Could you check a few things on this drawing? It's one solid part, dimensions in mm from its lowest x, y, z. Give positions to 0.01 mm unless a question says otherwise; leave off trailing zeros. Loops run counter-clockwise (first coordinate to the right, second up) from the corner with the lowest first, then second, coordinate; pieces in that order, holes last. Notation, with made-up numbers: (70, 15.25) - (118, 15.25) arc R32 ccw to (118, 45.25) - close; hole circle Ø1 at (86, -8). An arc over 180 degrees is marked (long way). Return JSON: item names as keys, results as strings. Group by question number.
(1) If we section it at B-B (x = 30): Please give me the cut outline in (y, z), then the cut area to 3 significant figures.
(2) If we mould it in two halves opening along Z, with no side actions, what happens to the marked faces 1, 2 and 3? For each: released by +Z, released by -Z, zero draft, split by the parting line, or undercut.
(3) I need wall thicknesses on probe 1 along Z at (x, y) = (118.5, 24); probe 2 along X at (y, z) = (9.25, 6.5) (1 decimal). Which ranges of each line are inside material? Lowest first, please. Write a range as [from, to].
(4) For P1, Ø6.5, axis at x = 74, y = 8.5, coming from the -Z side, with a flat end and sliding along its axis, tell me the tip position at first contact or that it passes through.
(5) If we section it at C-C (x = 69.85): State how many separate pieces and enclosed holes the cut face has, then the cut area to 3 significant figures.
(6) If we section it at A-A (z = 115.5): Please give me the cut outline in (x, y), then the cut area to 3 significant figures.
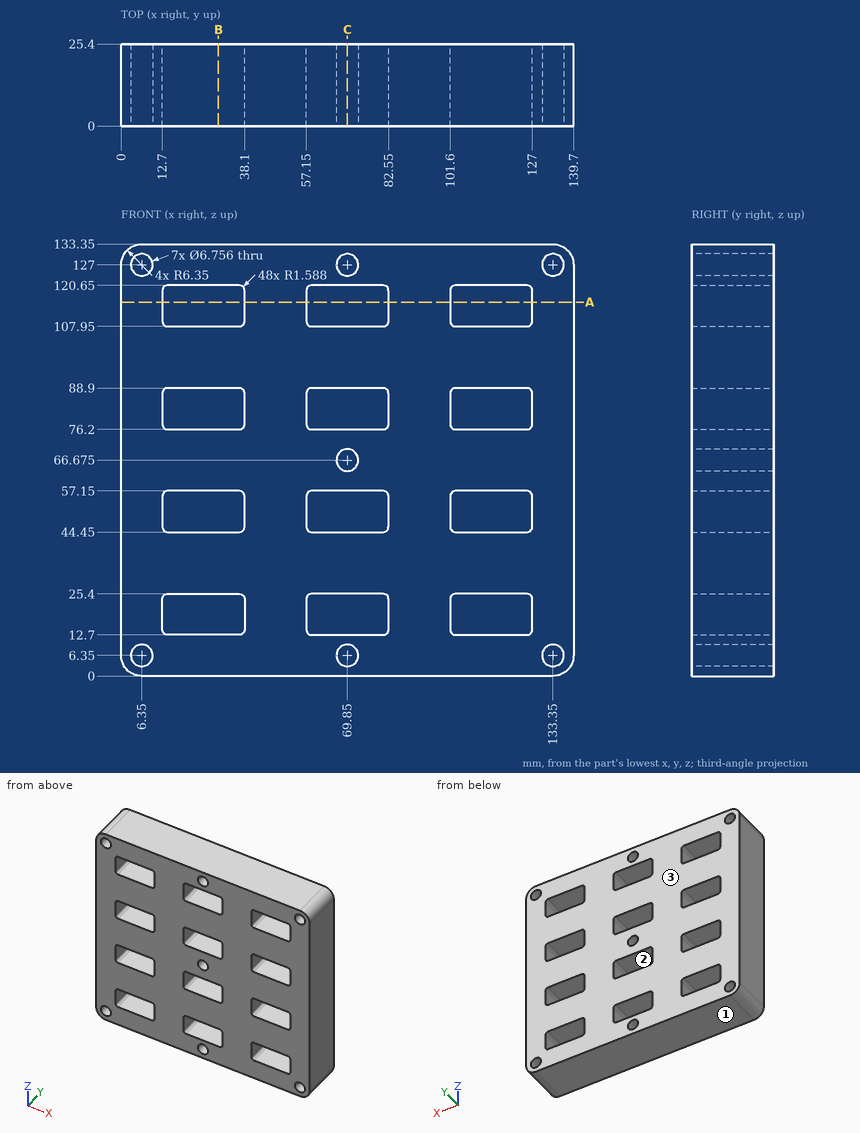
Values:
{
 "1": {"outline": "(0, 0) - (25.4, 0) - (25.4, 12.7) - (0, 12.7) - close; (0, 25.4) - (25.4, 25.4) - (25.4, 44.45) - (0, 44.45) - close; (0, 57.15) - (25.4, 57.15) - (25.4, 76.2) - (0, 76.2) - close; (0, 88.9) - (25.4, 88.9) - (25.4, 107.95) - (0, 107.95) - close; (0, 120.65) - (25.4, 120.65) - (25.4, 133.35) - (0, 133.35) - close", "area": "2,100 mm2"},
 "2": {"face 1": "released by -Z", "face 2": "undercut", "face 3": "zero draft"},
 "3": {"probe 1": "[0, 12.7], [25.4, 44.45], [57.15, 76.2], [88.9, 107.95], [120.65, 133.35]", "probe 2": "[0, 3], [9.7, 66.5], [73.2, 130], [136.7, 139.7]"},
 "4": {"P1": "z = 0"},
 "5": {"separate pieces": "8", "enclosed holes": "0", "area": "1,580 mm2"},
 "6": {"outline": "(0, 0) - (12.7, 0) - (12.7, 25.4) - (0, 25.4) - close; (38.1, 0) - (57.15, 0) - (57.15, 25.4) - (38.1, 25.4) - close; (82.55, 0) - (101.6, 0) - (101.6, 25.4) - (82.55, 25.4) - close; (127, 0) - (139.7, 0) - (139.7, 25.4) - (127, 25.4) - close", "area": "1,610 mm2"}
}
